Check sheet for the drawn part. Datum: minimum x, y, z corner. Units: mm. A direction names the side the tool comes from. Coordinates: 2 decimals unless noted, no trailing zeros. Write each loop counter-clockwise with the first axis right and the second up, starting at its lowest first coordinate (ties: lowest second). Pieces come first, ordered by that corner, then holes. Notation, with made-up numbers: M 10.25,66.25 L 34.25,66.25 A21 ccw 34.25,81.25 Z; hole C 84,53.5 d6. An arc over 180 degrees is marked long. Answer as a JSON object with one key per item and string values. Group by question number.
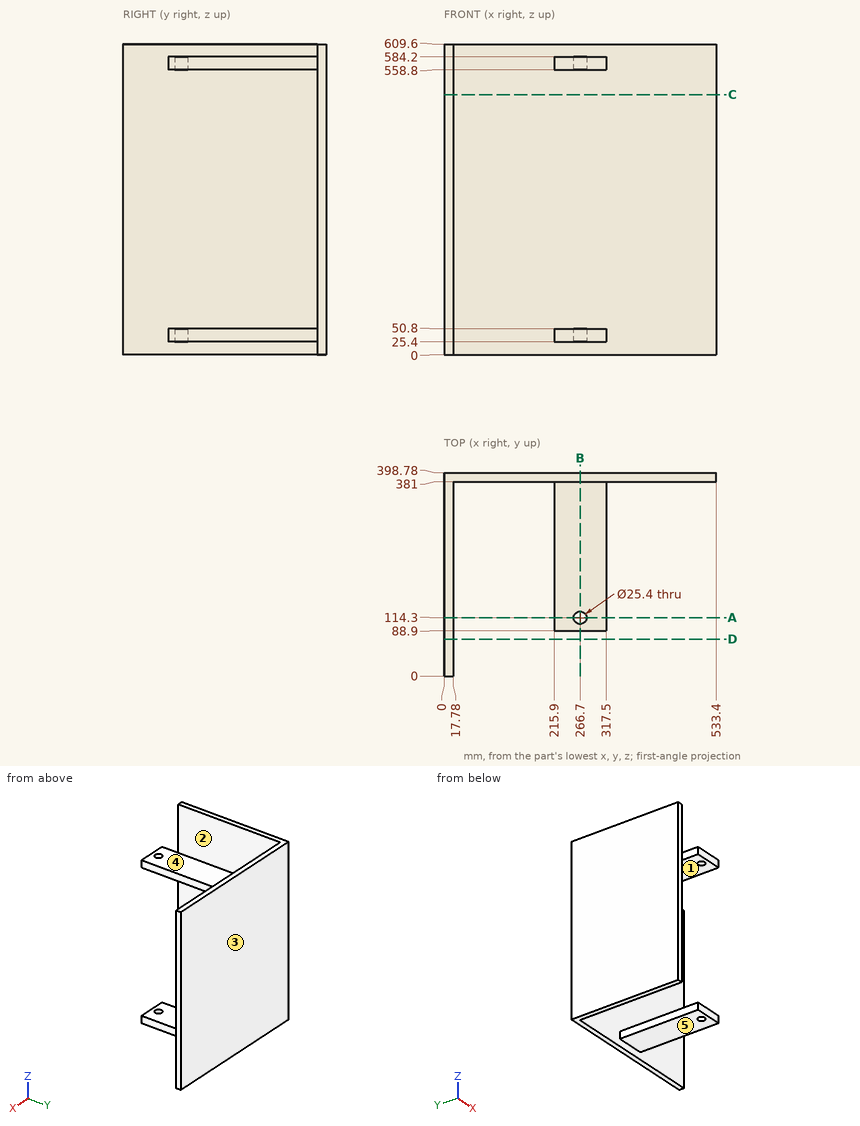
1) Set-up check for the marked faces 1, 2, 3, 4 and 5: record each of +Z, -Z, +X, -X, +Y, -Y from which the full face is reachable in a straight line by a thin tool's end or side.
2) Go/stop test with flat-tipped pins: pin 1 Ø7.5 at (y, z) = (223, 567.5) entering from +X; pin 2 Ø8 at (x, z) = (219.5, 544) entering from -Y; pin 3 Ø12 at (y, z) = (341.5, 106.5) entering from +X. Record where each tip stops, or that it passes through.
3) Material ranges on probe 1 along X at (y, z) = (114, 578); probe 2 along Z at (x, y) = (263, 277); probe 3 along Y at (x, z) = (266.7, 32.5), recorded low to high. Write a range as [from, to].
4) Section check C-C (z = 510.5). Record the cut outline in (x, y).
5) Section check A-A (y = 114.3). Record the cut outline in (x, z), then the cut area to 3 significant figures.
6) Section check B-B (x = 266.7). Record the cut outline in (y, z).
7) Section check D-D (y = 72.5). Record the cut outline in (x, z), then the cut area to 3 significant figures.
Entries:
{
 "1": {"face 1": "+X, -Y", "face 2": "+Z, -Z, -Y", "face 3": "+Z, -Z, +X, -X, +Y", "face 4": "+Z, +X, -Y", "face 5": "-Z, +X, -Y"},
 "2": {"pin 1": "x = 317.5", "pin 2": "y = 381", "pin 3": "x = 17.78"},
 "3": {"probe 1": "[0, 17.78], [215.9, 254], [279.4, 317.5]", "probe 2": "[25.4, 50.8], [558.8, 584.2]", "probe 3": "[88.9, 101.6], [127, 398.78]"},
 "4": {"outline": "M 0,0 L 17.78,0 L 17.78,381 L 533.4,381 L 533.4,398.78 L 0,398.78 Z"},
 "5": {"outline": "M 0,0 L 17.78,0 L 17.78,609.6 L 0,609.6 Z; M 215.9,25.4 L 254,25.4 L 254,50.8 L 215.9,50.8 Z; M 215.9,558.8 L 254,558.8 L 254,584.2 L 215.9,584.2 Z; M 279.4,25.4 L 317.5,25.4 L 317.5,50.8 L 279.4,50.8 Z; M 279.4,558.8 L 317.5,558.8 L 317.5,584.2 L 279.4,584.2 Z", "area": "14,700 mm^2"},
 "6": {"outline": "M 88.9,25.4 L 101.6,25.4 L 101.6,50.8 L 88.9,50.8 Z; M 88.9,558.8 L 101.6,558.8 L 101.6,584.2 L 88.9,584.2 Z; M 127,25.4 L 381,25.4 L 381,0 L 398.78,0 L 398.78,609.6 L 381,609.6 L 381,584.2 L 127,584.2 L 127,558.8 L 381,558.8 L 381,50.8 L 127,50.8 Z"},
 "7": {"outline": "M 0,0 L 17.78,0 L 17.78,609.6 L 0,609.6 Z", "area": "10,800 mm^2"}
}
